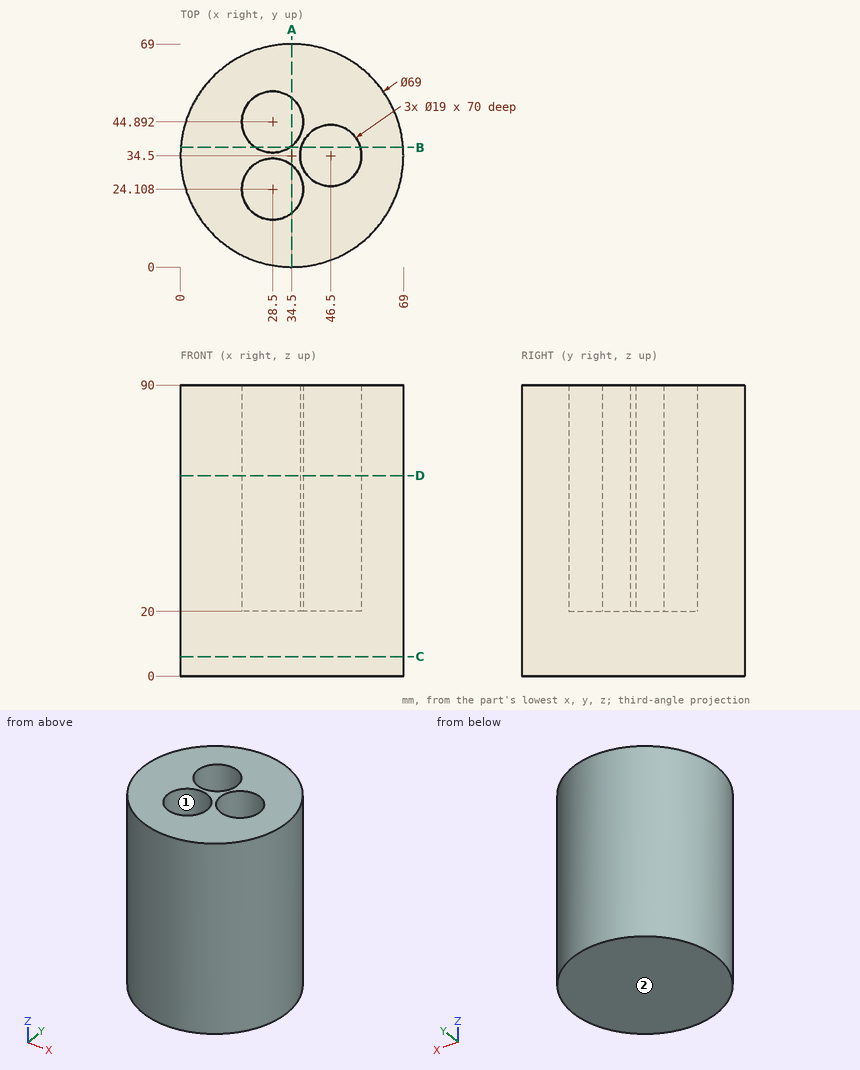
Could you check a few things on this drawing? It's one solid part, dimensions in mm from its lowest x, y, z. A direction names the side the tool comes from. Coordinates: 2 decimals unless noted, no trailing zeros. Order: outer loops, then holes, each group sorted by start corner. A loop starts at its lowest first (then second) coordinate and runs counter-clockwise, first axis right, second up. Notation, with made-up numbers: M 86,11.5 L 137,11.5 A3 ccw 137,15.5 Z; hole C 77.5,61 d3. An arc over 180 degrees is marked long. Use one line per item in the form item = value. Start each with the question number.
1. Suppose I cut it at D-D on z = 62. Write out the boundary of the cut face in (x, y), then the cut area to 3 significant figures.
2. Suppose I cut it at C-C on z = 6. Write out the boundary of the cut face in (x, y).
3. For pin 1 (1 mm diameter, centred on x = 10, z = 73, fed in from +Y) (1 decimal); pin 2 (5 mm diameter, centred on y = 25.5, z = 54, fed in from +X); pin 3 (3 mm diameter, centred on y = 43, z = 49.5, fed in from +X), each with a flat end and sliding along its axis, tell me the tip position at first contact or that it passes through.
4. Suppose I cut it at A-A on x = 34.5. Write out the boundary of the cut face in (y, z), then the cut area to 3 significant figures.
5. Suppose I cut it at B-B on y = 37. Write out the boundary of the cut face in (x, z) (1 decimal).
6. Please list where these lines run through material, in increasing order: line 1 (Y direction, x = 28.5, z = 46) (1 decimal); line 2 (Y direction, x = 28, z = 72) (1 decimal); line 3 (X direction, y = 34, z = 54).
7. On a 3-axis mill with a long thin cutter (end or side, diameter ignored), from which of +Z, -Z, +X, -X, +Y, -Y can I reach the whole of each face in a straight line? I mean the marked faces 1 and 2. Say none if no direction works.
Geometry says:
q1.outline = C 34.5,34.5 d69; hole C 28.5,24.11 d19; hole C 28.5,44.89 d19; hole C 46.5,34.5 d19
q1.area = 2,890 mm^2
q2.outline = C 34.5,34.5 d69
q3.pin_1 = 59.3
q3.pin_2 = 68.38
q3.pin_3 = 68.28
q4.outline = M 0,0 L 69,0 L 69,90 L 52.26,90 L 52.26,20 L 37.53,20 L 37.53,90 L 31.47,90 L 31.47,20 L 16.74,20 L 16.74,90 L 0,90 Z
q4.area = 4,150 mm^2
q5.outline = M 0.1,0 L 68.9,0 L 68.9,90 L 55.7,90 L 55.7,20 L 37.3,20 L 37.3,90 L 33.8,90 L 33.8,20 L 23.2,20 L 23.2,90 L 0.1,90 Z
q6.line_1 = 0.5 to 14.6, 33.6 to 35.4, 54.4 to 68.5
q6.line_2 = 0.6 to 14.6, 33.6 to 35.4, 54.4 to 68.4
q6.line_3 = 0 to 37.01, 55.99 to 69
q7.face_1 = +Z
q7.face_2 = -Z, +X, -X, +Y, -Y
